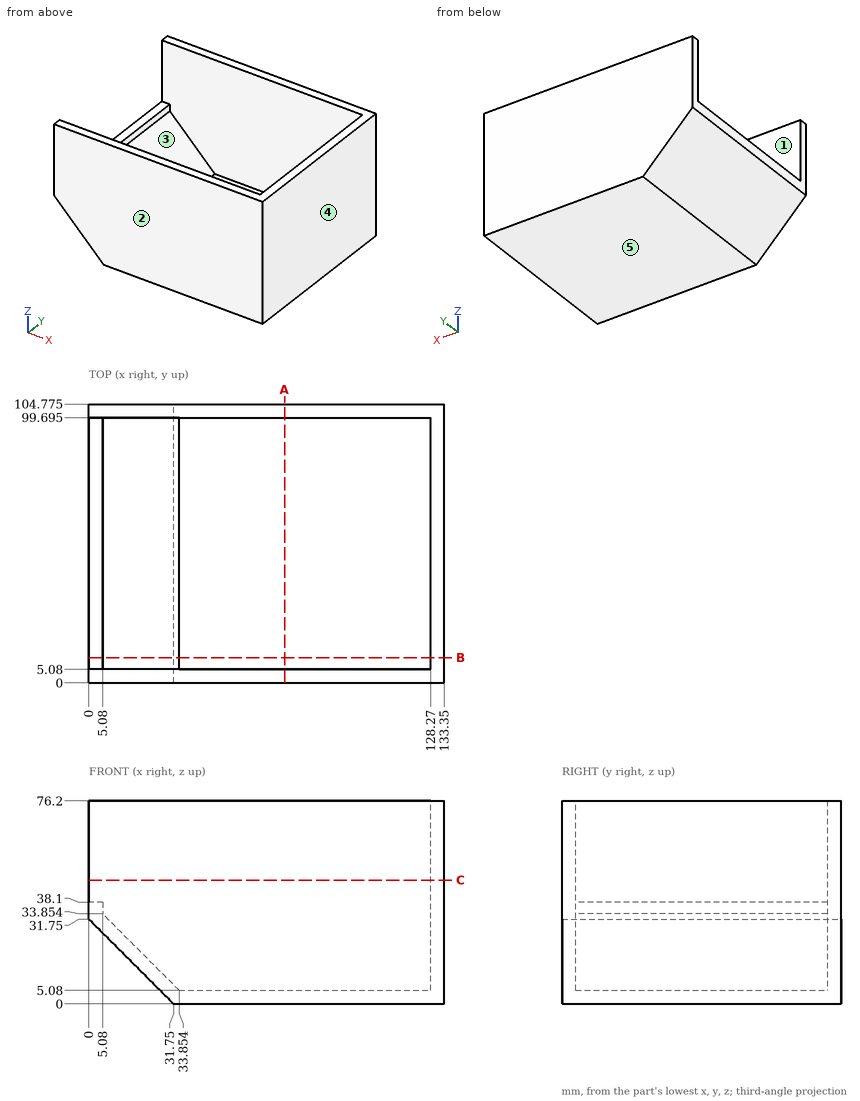
Source: three-view drawing plus pictorial views. Frame: mm from the lowest corner of the part. A direction names the side the tool comes from. Coordinates: 2 decimals unless noted, no trailing zeros. Order: outer loops, then holes, each group sorted by start corner. A loop starts at its lowest first (then second) coordinate and runs counter-clockwise, first axis right, second up. Notation, with made-up numbers: M 22,88 L 26,88 A22 cw 26,94 Z; hole C -40,60.5 d11. An arc over 180 degrees is marked long. One line per question, with ' | ' between items. Start each with the question number.
Item 1: Cut plane B-B, the plane y = 9.5. Return the cut outline in (x, z), then the cut area to 3 significant figures.
Item 2: Ray query, probe 1 along Y at (x, z) = (42.5, 66) (3 decimals); probe 2 along X at (y, z) = (69.5, 36); probe 3 along X at (y, z) = (55.5, 72). Return the intervals inside material, ascending. Write a range as [from, to].
Item 3: Cut plane C-C, the plane z = 46.5. Return the cut outline in (x, y) (3 decimals).
Item 4: Draft query along X for the marked faces 3, 4 and 5. Return one class per face: released by +X, released by -X, zero draft, split by the parting line, or undercut.
Item 5: Set-up query: the marked faces 1 and 2. Return all of +Z, -Z, +X, -X, +Y, -Y with unobstructed straight access to the full face (end or side cutting, diameter ignored); none if empty.
Item 6: Cut plane A-A, the plane x = 73.5. Return the cut outline in (y, z) (3 decimals), then the cut area to 4 significant figures.
Item 7: Pin query (flat end, axial travel): pin 1 Ø5.5 at (x, y) = (2.5, 48.5) entering from +Z; pin 2 Ø12 at (x, z) = (97.5, 51) entering from -Y; pin 3 Ø5 at (y, z) = (67, 48) entering from -X; pin 4 Ø3 at (x, y) = (111, 77.5) entering from +Z. Return the tip coordinate at first contact, or that it passes through.
A:
1) outline: M 0,31.75 L 31.75,0 L 133.35,0 L 133.35,76.2 L 128.27,76.2 L 128.27,5.08 L 33.85,5.08 L 5.08,33.85 L 5.08,38.1 L 0,38.1 Z | area: 1,120 mm2
2) probe 1: y = [0, 5.08], [99.695, 104.775] | probe 2: x = [0, 5.08], [128.27, 133.35] | probe 3: x = [128.27, 133.35]
3) outline: M 0,0 L 133.35,0 L 133.35,104.775 L 0,104.775 L 0,99.695 L 128.27,99.695 L 128.27,5.08 L 0,5.08 Z
4) face 3: undercut | face 4: released by +X | face 5: zero draft
5) face 1: +Z | face 2: +Z, -Z, +X, -X, -Y
6) outline: M 0,0 L 104.775,0 L 104.775,76.2 L 99.695,76.2 L 99.695,5.08 L 5.08,5.08 L 5.08,76.2 L 0,76.2 Z | area: 1,255 mm2
7) pin 1: stops at z = 38.1 | pin 2: stops at y = 0 | pin 3: stops at x = 128.27 | pin 4: stops at z = 5.08
